from build123d import *

# Parameters (mm, degrees)
BOSS_EXTRUDE1_DEPTH             = 22.5
M5X0_8_TAPPED_HOLE1_D           = 4.2
M5X0_8_TAPPED_HOLE1_DEPTH       = 12.0000014
M5X0_8_TAPPED_HOLE1_CSINK_D     = 5.05
M5X0_8_TAPPED_HOLE1_CSINK_ANGLE = 90
M5X0_8_TAPPED_HOLE1_TIP         = 1.2618073
CHAMFER1_SIZE                   = 3


with BuildPart() as part:
    # Sketch1 → Boss-Extrude1 (new body, symmetric)
    with BuildSketch(Plane.XY):
        with BuildLine():
            Line((-22.5, 20), (-22.5, 11))
            Line((-22.5, 11), (-21.792893219, 10.292893219))
            Line((-21.792893219, 10.292893219), (-21.792893219, -12.292893219))
            Line((-21.792893219, -12.292893219), (-21.085786438, -13))
            Line((-21.085786438, -13), (-8.900002224, -13))
            Line((-8.900002224, -13), (-5, -6.244997998))
            ThreePointArc((-5, -6.244997998), (0, 8), (5, -6.244997998))
            Line((5, -6.244997998), (8.900002224, -13))
            Line((8.900002224, -13), (21.085786438, -13))
            Line((21.085786438, -13), (21.792893219, -12.292893219))
            Line((21.792893219, -12.292893219), (21.792893219, 10.292893219))
            Line((21.792893219, 10.292893219), (22.5, 11))
            Line((22.5, 11), (22.5, 20))
            Line((22.5, 20), (9.5, 20))
            Line((9.5, 20), (8.792893219, 19.292893219))
            Line((8.792893219, 19.292893219), (-8.792893219, 19.292893219))
            Line((-8.792893219, 19.292893219), (-9.5, 20))
            Line((-9.5, 20), (-22.5, 20))
        make_face()
    extrude(amount=BOSS_EXTRUDE1_DEPTH, both=True)

    # M5x0.8 Tapped Hole1
    with Locations(Plane(origin=(16, 20, 16), x_dir=(0, 0, 1), z_dir=(0, 1, 0))):
        with Locations((0, 0), (-32, 0), (-32, -32), (0, -32)):
            CounterSinkHole(M5X0_8_TAPPED_HOLE1_D / 2, M5X0_8_TAPPED_HOLE1_CSINK_D / 2, depth=M5X0_8_TAPPED_HOLE1_DEPTH, counter_sink_angle=M5X0_8_TAPPED_HOLE1_CSINK_ANGLE)
            with Locations((0, 0, -(M5X0_8_TAPPED_HOLE1_DEPTH + M5X0_8_TAPPED_HOLE1_TIP / 2))):  # 118° drill point
                Cone(0, M5X0_8_TAPPED_HOLE1_D / 2, M5X0_8_TAPPED_HOLE1_TIP, mode=Mode.SUBTRACT)

    # Chamfer1
    chamfer1_edges = [part.edges().sort_by_distance(p)[0] for p in [
        (0, 8, -22.5),
        (0, 8, 22.5),
    ]]
    chamfer(chamfer1_edges, length=CHAMFER1_SIZE)


solid = part.part
CAD build for the part. Positions are in the model's coordinates, mm. A direction names the side the tool comes from. Coordinates: 2 decimals unless noted, no trailing zeros. Order: outer loops, then holes, each group sorted by start corner. A loop starts at its lowest first (then second) coordinate and runs counter-clockwise, first axis right, second up. Notation, with made-up numbers: (-33, 68) -> (-13, 68) arc R22 ccw to (-13, 107) -> close; hole circle Ø1 at (43.25, 11.5). An arc over 180 degrees is marked (long way). Answer in a Markdown table with one row per item.
1) Flat gauge pins, fed straight in: P1, Ø5.5, axis at x = 0, z = 0.5, coming from the +Y side; P2, Ø2.5, axis at x = -16, z = 16, coming from the +Y side; P3, Ø4, axis at x = -16, z = -16, coming from the +Y side. Where does each tip first touch, or does it go through?
Check values:
| item | result |
|---|---|
| P1 | y = 19.29 |
| P2 | y = 7.49 |
| P3 | y = 7.94 |
2) Band-saw the part on B-B (z = 3). List the corners of the cut face in (x, y) (3 decimals).
Check values:
| item | result |
|---|---|
| outline | (-22.5, 11) -> (-21.793, 10.293) -> (-21.793, -12.293) -> (-21.086, -13) -> (-8.9, -13) -> (-5, -6.245) arc R8 cw (long way) to (5, -6.245) -> (8.9, -13) -> (21.086, -13) -> (21.793, -12.293) -> (21.793, 10.293) -> (22.5, 11) -> (22.5, 20) -> (9.5, 20) -> (8.793, 19.293) -> (-8.793, 19.293) -> (-9.5, 20) -> (-22.5, 20) -> close |
3) Mould opens along X. For faces 1 (the face through (-15, -13, 0)), 2 (the face through (-22.5, 16, 0)), 3 (the face through (-6.977, -9.67, 0.315)) say: pulls with the +X half, pulls with the -X half, needs draft (parallel to the pull), parting line crosses it, or undercut.
Check values:
| item | result |
|---|---|
| face 1 | needs draft |
| face 2 | pulls with the -X half |
| face 3 | undercut |
4) Band-saw the part on D-D (x = 0). List the corners of the cut face in (y, z), and give its area (3 significant figures).
Check values:
| item | result |
|---|---|
| outline | (8, -19.5) -> (11, -22.5) -> (19.29, -22.5) -> (19.29, 22.5) -> (11, 22.5) -> (8, 19.5) -> close |
| area | 499 mm2 |
5) Band-saw the part on A-A (y = 0). List the corners of the cut face in (x, z), and give its area (3 significant figures).
Check values:
| item | result |
|---|---|
| outline | (-21.79, -22.5) -> (-11, -22.5) -> (-8, -19.5) -> (-8, 19.5) -> (-11, 22.5) -> (-21.79, 22.5) -> close; (8, -19.5) -> (11, -22.5) -> (21.79, -22.5) -> (21.79, 22.5) -> (11, 22.5) -> (8, 19.5) -> close |
| area | 1,220 mm2 |
6) Band-saw the part on C-C (y = 13). List the corners of the cut face in (x, z).
Check values:
| item | result |
|---|---|
| outline | (-22.5, -22.5) -> (22.5, -22.5) -> (22.5, 22.5) -> (-22.5, 22.5) -> close; hole circle Ø4.2 at (-16, -16); hole circle Ø4.2 at (-16, 16); hole circle Ø4.2 at (16, -16); hole circle Ø4.2 at (16, 16) |
7) Drill centre lines: line 1 (X direction, y = 13, z = -16); line 2 (X direction, y = 10, z = 16). Where is each one in solid material? Low to high.
Check values:
| item | result |
|---|---|
| line 1 | -22.5 to -18.1, -13.9 to 13.9, 18.1 to 22.5 |
| line 2 | -21.79 to -18.1, -13.9 to 13.9, 18.1 to 21.79 |
8) Which spindle directions (+Z, -Z, +X, -X, +Y, -Y) get a long thin tool onto all of the face, cutting with end or side? Do faces 4 (the face through (17.77, 13.71, 14.87)), 5 (the face through (6.923, -9.575, 0.315)), 6 (the face through (0, 19.293, 0)). Say none if no direction does.
Check values:
| item | result |
|---|---|
| face 4 | +Y |
| face 5 | +Z, -Z, -Y |
| face 6 | +Z, -Z, +Y |
